from build123d import *

# Parameters (mm, degrees)
F0_R          = 2
F3_DEPTH      = 2
F3_DEPTH_BACK = 2
F6_DEPTH      = 34


with BuildPart() as f1:
    # F0 (on Top) → F1 (revolve)
    with BuildSketch(Plane.XY):
        Circle(F0_R)
    revolve(axis=Axis((-18, 1.301999, 0), (0, 1, 0)))

    # F2 (on Front) → F3 (join, two sides)
    with BuildSketch(Plane.XZ) as f3_sk:
        Polygon((1.025022, 4), (-12.974978, 4), (-12.974978, -4), (-12.974978, -4.111864), (1.025022, -4.111864), align=None)
    extrude(amount=F3_DEPTH)
    extrude(f3_sk.sketch, amount=-F3_DEPTH_BACK)

    # F5 (on offset) → F6 (cut)
    with BuildSketch(Plane.YZ.offset(25)):
        Polygon((0, 0.5), (-2, 2), (-2, -2), (0, -0.5), (2, -2), (2, 2), align=None)
    extrude(amount=-F6_DEPTH, mode=Mode.SUBTRACT)


solid = f1.part
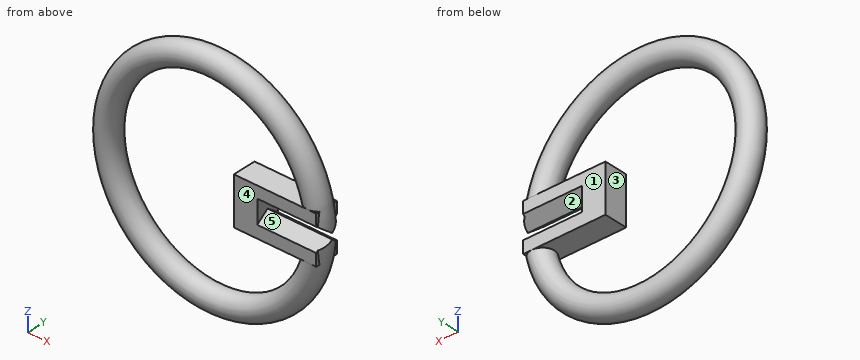
Read the model definition and answer for the solid it produces. Units are mm, in the model's axes. Face numbers are marked on the shaded views. A direction names the side the tool comes from. Round coordinates to 2 decimals unless told otherwise and drop trailing zeros. Loops run counter-clockwise (first coordinate to the right, second up) from the corner with the lowest first, then second, coordinate; pieces in that order, holes last.
Q1. Consider probe 1 along Z at (x, y) = (-10.5, 0.35); probe 2 along Z at (x, y) = (-11, 1.8); probe 3 along X at (y, z) = (0.7, -2.5). Determine where each line is inside the solid, lowest interval first.
Q2. Which of the six approach directions +Z, -Z, +X, -X, +Y, -Y give full straight-line access (tool end or side, diameter ignored) to the marked faces 3, 4 and 5?
Q3. Each of these flat-tipped pins is pushed along its axis until it touches: pin 1 (4 mm diameter, centred on x = -25, z = -11.5, fed in from +Y); pin 2 (1.2 mm diameter, centred on x = -4, y = -1, fed in from -Z); pin 3 (0.7 mm diameter, centred on y = 2, z = 2.5, fed in from +X) (3 decimals); pin 4 (0.7 mm diameter, centred on y = 1.5, z = -3, fed in from +X). Where does it stop, or does it pass through?
Q4. Section B-B on x = -8 is taken. Give the number of separate pieces and of enclosed holes in the cut face, and give its area (3 significant figures).
Q5. Determine the mould class of the marked faces 1 and 2 for opening direction Z: released by +Z, released by -Z, zero draft, split by the parting line, or undercut.
Q6. Section A-A on y = 0.65 is taken. Write down the section's boundary in (x, z).
Output:
1. probe 1: z = -18.51 to -14.17, -4.11 to 4, 14.17 to 18.51
1. probe 2: z = -17.53 to -15.63, -4.11 to 4, 15.63 to 17.53
1. probe 3: x = -37.72 to -33.93, -12.97 to 1.72
2. face 3: +Y, -Y
2. face 4: +Z, -Z, +X, -X, -Y
2. face 5: +X, -Y
3. pin 1: passes through
3. pin 2: stops at z = -14.6
3. pin 3: stops at x = 1.025
3. pin 4: stops at x = 1.41
4. separate pieces: 4
4. enclosed holes: 0
4. area: 52.8 mm2
5. face 1: zero draft
5. face 2: undercut
6. outline: (-9, -0.99) - (-9, 0.99) - (1.87, 0.99) arc R19.89 ccw (long way) to (1.87, -0.99) - close; hole (-12.97, -4.11) - (-12.97, 4) - (-2.4, 4) arc R16.11 ccw (long way) to (-2.43, -4.11) - close
